Geometry: final body of the model. Coordinates: model frame, mm. A direction names the side the tool comes from. Give positions to 0.01 mm unless a question says otherwise; leave off trailing zeros. Write each loop counter-clockwise with the first axis right and the second up, starting at its lowest first coordinate (ties: lowest second). Pieces come first, ordered by that corner, then holes.
from build123d import *
from build123d.topology import SkipClean

# Parameters (mm, degrees)
EXTRUDE_2_DEPTH     = 50
CUT_EXTRUDE_1_DEPTH = 52
SKETCH_3_R          = 62.5
EXTRUDE_3_DEPTH     = 1.5
EXTRUDE_START       = 5
EXTRUDE_5_DEPTH     = 5
EXTRUDE_6_DEPTH     = 47
CUT_EXTRUDE_2_DEPTH = 50
EXTRUDE_7_REACH     = 132.126
SKETCH_12_R         = 0.75
CUT_EXTRUDE_3_DEPTH = 5


with BuildPart() as part:
    # 草图1 → 凸台-拉伸2 (new body)
    # profile 1 of 3: a face of its own
    with BuildSketch(Plane.XY):
        Polygon((-3, -40.842640687), (-3, -47), (3.157359313, -47), align=None)
    # profile 2 of 3: a face of its own
    with BuildSketch(Plane.XY):
        Polygon((-3, -3.157359313), (3.157359313, 3), (40.842640687, 3), (47, -3.157359313), (47, -40.842640687), (40.842640687, -47), (3.157359313, -47), (-3, -40.842640687), align=None)
        Polygon((0, -39.6), (4.4, -44), (39.6, -44), (44, -39.6), (44, -4.4), (39.6, 0), (4.4, 0), (0, -4.4), align=None, mode=Mode.SUBTRACT)
    # profile 3 of 3: a face of its own
    with BuildSketch(Plane.XY):
        Polygon((47, -47), (40.842640687, -47), (47, -40.842640687), align=None)
    extrude(amount=EXTRUDE_2_DEPTH)

    # 草图2 → 切除-拉伸1 (cut)
    with BuildSketch(Plane.XY.offset(50)):
        with BuildLine():
            ThreePointArc((4.8, -45.5), (4.694427191, -45.052786405), (4.4, -44.7))
            Line((4.4, -44.7), (4.4, -46.3))
            ThreePointArc((4.4, -46.3), (4.694427191, -45.947213595), (4.8, -45.5))
        make_face()
        with BuildLine():
            Line((4.4, -46.3), (4.4, -44.7))
            ThreePointArc((4.4, -44.7), (2.8, -45.5), (4.4, -46.3))
        make_face()
        with BuildLine():
            ThreePointArc((4.8, -45.5), (4.694427191, -45.052786405), (4.4, -44.7))
            Line((4.4, -44.7), (4.4, -46.3))
            ThreePointArc((4.4, -46.3), (4.694427191, -45.947213595), (4.8, -45.5))
        make_face()
        with BuildLine():
            Line((4.4, -46.3), (4.4, -44.7))
            ThreePointArc((4.4, -44.7), (2.8, -45.5), (4.4, -46.3))
        make_face()
        with BuildLine():
            Line((39.6, -44), (4.4, -44))
            Line((4.4, -44), (4.4, -44.7))
            ThreePointArc((4.4, -44.7), (4.694427191, -45.052786405), (4.8, -45.5))
            ThreePointArc((4.8, -45.5), (4.694427191, -45.947213595), (4.4, -46.3))
            Line((4.4, -46.3), (4.4, -47))
            Line((4.4, -47), (39.6, -47))
            Line((39.6, -47), (39.6, -46.3))
            ThreePointArc((39.6, -46.3), (39.2, -45.5), (39.6, -44.7))
            Line((39.6, -44.7), (39.6, -44))
        make_face()
        with BuildLine():
            ThreePointArc((41.2, -45.5), (40.647213595, -44.605572809), (39.6, -44.7))
            Line((39.6, -44.7), (39.6, -46.3))
            ThreePointArc((39.6, -46.3), (40.647213595, -46.394427191), (41.2, -45.5))
        make_face()
        with BuildLine():
            Line((39.6, -46.3), (39.6, -44.7))
            ThreePointArc((39.6, -44.7), (39.2, -45.5), (39.6, -46.3))
        make_face()
        with BuildLine():
            ThreePointArc((41.2, -45.5), (40.647213595, -44.605572809), (39.6, -44.7))
            Line((39.6, -44.7), (39.6, -46.3))
            ThreePointArc((39.6, -46.3), (40.647213595, -46.394427191), (41.2, -45.5))
        make_face()
        with BuildLine():
            Line((39.6, -46.3), (39.6, -44.7))
            ThreePointArc((39.6, -44.7), (39.2, -45.5), (39.6, -46.3))
        make_face()
    extrude(amount=-CUT_EXTRUDE_1_DEPTH, mode=Mode.SUBTRACT)

    # 草图3 → 凸台-拉伸3 (add)
    with BuildSketch(Plane(origin=(0, 0, 0), x_dir=(-1, 0, 0), z_dir=(0, 0, -1))):
        with Locations((-22, -22)):
            Circle(SKETCH_3_R)
    extrude(amount=EXTRUDE_3_DEPTH)

    # 草图4 → 凸台-拉伸5 (add)
    with SkipClean():  # the faces are left unmerged after this step: merging them gives an invalid solid
        with BuildSketch(Plane.XY.offset(EXTRUDE_START)):
            with BuildLine():
                Line((-3, -79.282196187), (-3, -47))
                Line((-3, -47), (-3, -3.157359313))
                Line((-3, -3.157359313), (3.157359313, 3))
                Line((3.157359313, 3), (40.842640687, 3))
                Line((40.842640687, 3), (47, -3.157359313))
                Line((47, -3.157359313), (47, -4.4))
                Line((47, -4.4), (81.970742867, -4.4))
                ThreePointArc((81.970742867, -4.4), (-19.322802913, 24.890041154), (-3, -79.282196187))
            make_face()
            with BuildLine():
                Line((43.3, -47), (43.3, -80.758488748))
                ThreePointArc((43.3, -80.758488748), (65.929564348, -66.457208372), (80.5, -44))
                Line((80.5, -44), (47, -44))
                Line((47, -44), (47, -47))
                Line((47, -47), (43.3, -47))
            make_face()
        extrude(amount=-EXTRUDE_5_DEPTH)

    # 草图8 → 凸台-拉伸6 (add)
    with SkipClean():  # the faces are left unmerged after this step: merging them gives an invalid solid
        with BuildSketch(Plane.XY.offset(50)):
            Polygon((47, 3), (47, -3.157359313), (40.842640687, 3), align=None)
        extrude(amount=-EXTRUDE_6_DEPTH)

    # 草图9 → 切除-拉伸2 (cut)
    with SkipClean():  # the faces are left unmerged after this step: merging them gives an invalid solid
        with BuildSketch(Plane.XY.offset(50)):
            with BuildLine():
                Line((44, -4.4), (44, -39.6))
                Line((44, -39.6), (44.7, -39.6))
                ThreePointArc((44.7, -39.6), (45.5, -39.2), (46.3, -39.6))
                Line((46.3, -39.6), (47, -39.6))
                Line((47, -39.6), (47, -4.4))
                Line((47, -4.4), (46.3, -4.4))
                ThreePointArc((46.3, -4.4), (45.5, -4.8), (44.7, -4.4))
                Line((44.7, -4.4), (44, -4.4))
            make_face()
            with BuildLine():
                ThreePointArc((46.5, -3.8), (45.183772234, -2.851316702), (44.7, -4.4))
                Line((44.7, -4.4), (46.3, -4.4))
                ThreePointArc((46.3, -4.4), (46.448683298, -4.116227766), (46.5, -3.8))
            make_face()
            with BuildLine():
                Line((46.3, -4.4), (44.7, -4.4))
                ThreePointArc((44.7, -4.4), (45.5, -4.8), (46.3, -4.4))
            make_face()
            with BuildLine():
                ThreePointArc((46.5, -3.8), (45.183772234, -2.851316702), (44.7, -4.4))
                Line((44.7, -4.4), (46.3, -4.4))
                ThreePointArc((46.3, -4.4), (46.448683298, -4.116227766), (46.5, -3.8))
            make_face()
            with BuildLine():
                Line((46.3, -4.4), (44.7, -4.4))
                ThreePointArc((44.7, -4.4), (45.5, -4.8), (46.3, -4.4))
            make_face()
            with BuildLine():
                ThreePointArc((46.3, -39.6), (45.5, -39.2), (44.7, -39.6))
                Line((44.7, -39.6), (46.3, -39.6))
            make_face()
            with BuildLine():
                Line((46.3, -39.6), (44.7, -39.6))
                ThreePointArc((44.7, -39.6), (45.183772234, -41.148683298), (46.5, -40.2))
                ThreePointArc((46.5, -40.2), (46.448683298, -39.883772234), (46.3, -39.6))
            make_face()
            with BuildLine():
                ThreePointArc((46.3, -39.6), (45.5, -39.2), (44.7, -39.6))
                Line((44.7, -39.6), (46.3, -39.6))
            make_face()
            with BuildLine():
                Line((46.3, -39.6), (44.7, -39.6))
                ThreePointArc((44.7, -39.6), (45.183772234, -41.148683298), (46.5, -40.2))
                ThreePointArc((46.5, -40.2), (46.448683298, -39.883772234), (46.3, -39.6))
            make_face()
        extrude(amount=-CUT_EXTRUDE_2_DEPTH, mode=Mode.SUBTRACT)

    # 草图11 → 凸台-拉伸7 (add, up to next)
    with BuildSketch(Plane.XY.offset(50), mode=Mode.PRIVATE) as extrude_7_sk1:
        Polygon((-3, 3), (3.157359313, 3), (-3, -3.157359313), align=None)
    extrude_7_tool1 = extrude(extrude_7_sk1.sketch, amount=-EXTRUDE_7_REACH, mode=Mode.PRIVATE) - part.part
    add(extrude_7_tool1.solids().sort_by_distance((-0.947547, 0.947547, 50))[0])

    # 草图12 → 切除-拉伸3 (cut)
    with SkipClean():  # the faces are left unmerged after this step: merging them gives an invalid solid
        with BuildSketch(Plane.XY.offset(50)):
            Circle(SKETCH_12_R)
            with Locations((44, 0)):
                Circle(SKETCH_12_R)
            with Locations(Location((0, -44, 0), (0, 0, 180))):
                Circle(SKETCH_12_R)
            with Locations(Location((44, -44, 0), (0, 0, 180))):
                Circle(SKETCH_12_R)
        extrude(amount=-CUT_EXTRUDE_3_DEPTH, mode=Mode.SUBTRACT)

    # 草图14 → 放样3 section 0
    with SkipClean():  # the faces are left unmerged after this step: merging them gives an invalid solid
        with BuildSketch(Plane.XY.offset(50)):
            with BuildLine():
                Line((43.3, -47), (47, -47))
                Line((47, -47), (47, -48))
                Line((47, -48), (43.3, -48))
                Line((43.3, -48), (43.3, -47))
            make_face()
        # 草图13 → 放样3 section 1
        with BuildSketch(Plane.XY.offset(5)):
            with BuildLine():
                Line((47, -47), (43.3, -47))
                Line((43.3, -47), (43.3, -77))
                Line((43.3, -77), (47, -77))
                Line((47, -77), (47, -47))
            make_face()
        loft()

    # 草图15 → 放样4 section 0
    with SkipClean():  # the faces are left unmerged after this step: merging them gives an invalid solid
        with BuildSketch(Plane.XY.offset(5)):
            with BuildLine():
                Line((47, -44), (77, -44))
                Line((77, -44), (77, -48))
                Line((77, -48), (47, -48))
                Line((47, -48), (47, -44))
            make_face()
        # 草图16 → 放样4 section 1
        with BuildSketch(Plane.XY.offset(50)):
            with BuildLine():
                Line((47, -48), (48, -48))
                Line((48, -48), (48, -44))
                Line((48, -44), (47, -44))
                Line((47, -44), (47, -48))
            make_face()
        loft()

    # 草图18 → 放样5 section 0
    with SkipClean():  # the faces are left unmerged after this step: merging them gives an invalid solid
        with BuildSketch(Plane.XY.offset(50)):
            with BuildLine():
                Line((-3, 3), (-4, 3))
                Line((-4, 3), (-4, -2))
                Line((-4, -2), (-3, -2))
                Line((-3, -2), (-3, 3))
            make_face()
        # 草图17 → 放样5 section 1
        with BuildSketch(Plane.XY.offset(5)):
            with BuildLine():
                Line((-3, 3), (-33, 3))
                Line((-33, 3), (-33, -2))
                Line((-33, -2), (-3, -2))
                Line((-3, -2), (-3, 3))
            make_face()
        loft()

    # 草图20 → 放样6 section 0
    with SkipClean():  # the faces are left unmerged after this step: merging them gives an invalid solid
        with BuildSketch(Plane.XY.offset(50)):
            with BuildLine():
                Line((42, 3), (47, 3))
                Line((47, 3), (47, 4))
                Line((47, 4), (42, 4))
                Line((42, 4), (42, 3))
            make_face()
        # 草图19 → 放样6 section 1
        with BuildSketch(Plane.XY.offset(5)):
            with BuildLine():
                Line((47, 3), (42, 3))
                Line((42, 3), (42, 33))
                Line((42, 33), (47, 33))
                Line((47, 33), (47, 3))
            make_face()
        loft()

    # 草图22 → 放样7 section 0
    with SkipClean():  # the faces are left unmerged after this step: merging them gives an invalid solid
        with BuildSketch(Plane.XY.offset(50)):
            with BuildLine():
                Line((-3, -47), (-4, -47))
                Line((-4, -47), (-4, -42))
                Line((-4, -42), (-3, -42))
                Line((-3, -42), (-3, -47))
            make_face()
        # 草图21 → 放样7 section 1
        with BuildSketch(Plane.XY.offset(5)):
            with BuildLine():
                Line((-3, -47), (-33, -47))
                Line((-33, -47), (-33, -42))
                Line((-33, -42), (-3, -42))
                Line((-3, -42), (-3, -47))
            make_face()
        loft()

    # 草图24 → 放样9 section 0
    with SkipClean():  # the faces are left unmerged after this step: merging them gives an invalid solid
        with BuildSketch(Plane.XY.offset(50)):
            with BuildLine():
                Line((-3, 3), (2, 3))
                Line((2, 3), (2, 4))
                Line((2, 4), (-3, 4))
                Line((-3, 4), (-3, 3))
            make_face()
        # 草图23 → 放样9 section 1
        with BuildSketch(Plane.XY.offset(5)):
            with BuildLine():
                Line((-3, 3), (2, 3))
                Line((2, 3), (2, 33))
                Line((2, 33), (-3, 33))
                Line((-3, 33), (-3, 3))
            make_face()
        loft()


solid = part.part
Q1. Pull-direction query (X, two-part tool) for faces 4 (the flat face through (2.2, -2.2, 24.6)), 5 (the flat face through (47, -1, 27)), 6 (the flat face through (45.176, -62.703, 27.185)); classes: released by +X, released by -X, zero draft, split by the parting line, or undercut.
Filled sheet:
face 4: undercut
face 5: released by +X
face 6: zero draft
Q2. Section A-A on x = 22. Output: boundary loops of the cut face in (y, z).
Filled sheet:
outline: (-84.5, -1.5) - (40.5, -1.5) - (40.5, 5) - (3, 5) - (3, 50) - (0, 50) - (0, 0) - (-84.5, 0) - close
Q3. Pin query (flat end, axial travel): P1, Ø0.9, axis at x = 0, y = 0, coming from the +Z side; P2, Ø2.5, axis at x = 46, y = -29, coming from the +Z side; P3, Ø1, axis at x = 6.5, z = 30, coming from the +Y side. Return the tip coordinate at first contact, or that it passes through.
Filled sheet:
P1: stops at z = 45
P2: stops at z = 0
P3: stops at y = 3
Q4. Access query for faces 1 (the flat face through (2.2, -41.8, 24.6)), 2 (the flat face through (-3, -63, 3)), 3 (the flat face through (60.1, -4.4, 4.7)). Directions: +Z, -Z, +X, -X, +Y, -Y. A direction counts if a zero-diameter tool reaches every point of the face in a straight line with its end or side. Return the directions, or none.
Filled sheet:
face 1: +Z
face 2: +Z, -Y
face 3: +Z, +X
Q5. Ray query, line 1 along Y through (x, z) = (44, 48); line 2 along X through (y, z) = (-40.2, 28.5); line 3 along Y through (x, z) = (3, 15). Return the intervals inside material, ascending.
Filled sheet:
line 1: y = -49.29 to -44.75, -43.25 to -39.6, -4.4 to -0.75, 0.75 to 5.29
line 2: x = -3 to 0.6, 43.4 to 44.5, 46.5 to 47
line 3: y = -47 to -46.1, -44.9 to -42.6, -1.4 to 3
